from build123d import *

# Parameters (mm, degrees)
SKETCH1_W           = 18
SKETCH1_H           = 25
BOSS_EXTRUDE1_DEPTH = 18
SKETCH2_W           = 7
SKETCH2_H           = 12.4
CUT_EXTRUDE1_DEPTH  = 20
BOSS_EXTRUDE2_DEPTH = 100
CUT_EXTRUDE2_DEPTH  = 100


with BuildPart() as part:
    # Sketch1 → Boss-Extrude1 (new body)
    with BuildSketch(Plane(origin=(0, 0, 0), x_dir=(0, 0, -1), z_dir=(1, 0, 0))):
        Rectangle(SKETCH1_W, SKETCH1_H)
    extrude(amount=BOSS_EXTRUDE1_DEPTH)

    # Sketch2 → Cut-Extrude1 (cut)
    with BuildSketch(Plane.XZ.offset(12.5)):
        with Locations((12, 0)):
            Rectangle(SKETCH2_W, SKETCH2_H)
    extrude(amount=-CUT_EXTRUDE1_DEPTH, mode=Mode.SUBTRACT)

    # Sketch3 → Boss-Extrude2 (add)
    with BuildSketch(Plane(origin=(0, 12.5, 0), x_dir=(1, 0, 0), z_dir=(0, 1, 0))):
        with BuildLine():
            Line((0, 5.656854249), (0, -5.656854249))
            ThreePointArc((0, -5.656854249), (16, 0), (0, 5.656854249))
        make_face()
    extrude(amount=BOSS_EXTRUDE2_DEPTH)

    # Sketch6 → Revolve2 (revolve)
    with BuildSketch(Plane(origin=(0, 112.5, 0), x_dir=(1, 0, 0), z_dir=(0, 1, 0))):
        with BuildLine():
            Line((8, 15), (8, -15))
            ThreePointArc((8, -15), (-7, 0), (8, 15))
        make_face()
    revolve(axis=Axis((8, 112.5, -15), (0, 0, 1)))

    # Sketch7 → Cut-Extrude2 (cut)
    with BuildSketch(Plane.ZY):
        with BuildLine():
            ThreePointArc((-5.656854249, 101.142183308), (0, 203.728611238), (5.656854249, 101.142183308))
            ThreePointArc((5.656854249, 101.142183308), (0, 99.81142246), (-5.656854249, 101.142183308))
        make_face()
    extrude(amount=CUT_EXTRUDE2_DEPTH, mode=Mode.SUBTRACT)


solid = part.part
Work out the finished part from the listing and answer in its coordinate system (mm). A direction names the side the tool comes from. Give positions to 0.01 mm unless a question says otherwise; leave off trailing zeros. Write each loop counter-clockwise with the first axis right and the second up, starting at its lowest first coordinate (ties: lowest second). Pieces come first, ordered by that corner, then holes.
Q1. Given pin 1 (13.5 mm diameter, centred on y = -1, z = 1.5, fed in from +X); pin 2 (5.5 mm diameter, centred on x = 13.5, z = 4.5, fed in from +Y); pin 3 (1.7 mm diameter, centred on x = 4.5, z = -6.5, fed in from +Y), each flat-ended and moving along its own axis, determine where each tip first touches the part or whether it passes through.
Answer:
pin 1: stops at x = 18
pin 2: stops at y = 126.85
pin 3: stops at y = 126
Q2. The part is cut by section B-B on x = 11.75. Give the vertices of the cut face in (y, z).
Answer:
outline: (-12.5, -9) - (12.5, -9) - (12.5, -7.64) - (100.15, -7.64) arc R14.52 ccw (long way) to (100.15, 7.64) - (12.5, 7.64) - (12.5, 9) - (-12.5, 9) - (-12.5, 6.2) - (7.5, 6.2) - (7.5, -6.2) - (-12.5, -6.2) - close
Q3. A tool of negligible diameter and unlimited length cuts with its end or side. For faces 4 (the face through (9, 0, -9)), 5 (the face through (9, 0, 9)), 6 (the face through (12, -3, 6.2)), 7 (the face through (17, 12.5, -1)), 8 (the face through (2, 12.5, 8)), from which of +Z, -Z, +X, -X, +Y, -Y can it reach the whole face along a straight path? Write none if from no direction.
Answer:
face 4: -Z, +X, -X, -Y
face 5: +Z, +X, -X, -Y
face 6: -Y
face 7: +X
face 8: +Z, -X
Q4. The part is cut by section A-A on z = 0. Give the vertices of the cut face in (x, y), and give its area (3 significant figures).
Answer:
outline: (0, -12.5) - (8.5, -12.5) - (8.5, 7.5) - (15.5, 7.5) - (15.5, -12.5) - (18, -12.5) - (18, 12.5) - (16, 12.5) - (16, 99.81) arc R15 ccw to (0, 125.19) - close
area: 2,260 mm2
Q5. The part is cut by section C-C on y = 17. Give the vertices of the cut face in (x, z), and give its area (3 significant figures).
Answer:
outline: (0, -5.66) arc R9 ccw (long way) to (0, 5.66) - close
area: 239 mm2
Q6. Straight lines are drawn through the part: L1, parallel to X at y = 4.5, z = 4.5; L2, parallel to Y at x = 3, z = -8.75; L3, parallel to X at y = -2.5, z = 6.75. For each, find the intervals that lie inside material, in ascending order.
Answer:
L1: x = 0 to 8.5, 15.5 to 18
L2: y = -12.5 to 12.5, 101.39 to 123.61
L3: x = 0 to 18
Q7. The part is cut by section D-D on x = 20. Give the vertices of the cut face in (y, z).
Answer:
outline: circle Ø18 at (112.5, 0)
Q8. For a pull along Z with two mould halves and no side action, classify faces 1 (the face through (12, -3, -6.2)), 2 (the face through (16, 56, 0)), 3 (the face through (2, 12.5, -8)) as released by +Z, released by -Z, zero draft, split by the parting line, or undercut.
Answer:
face 1: undercut
face 2: split by the parting line
face 3: zero draft
